Read the model definition and answer for the solid it produces. Units are mm, in the model's axes. A direction names the side the tool comes from. Round coordinates to 2 decimals unless told otherwise and drop trailing zeros. Loops run counter-clockwise (first coordinate to the right, second up) from the corner with the lowest first, then second, coordinate; pieces in that order, holes last. Notation, with made-up numbers: (56.5, -9) -> (81.5, -9) arc R22 cw to (81.5, 7) -> close; hole circle Ø7 at (66.5, -14.75). An arc over 180 degrees is marked (long way). Put each result on its own line as item: value.
from build123d import *

# Parameters (mm, degrees)
SKETCH1_W          = 30
SKETCH1_H          = 75
BASE_FLANGE1_DEPTH = 0.67
EDGE_FLANGE1_DEPTH = 75
SKETCH7_R          = 1.7
CUT_EXTRUDE1_DEPTH = 10
FILLET1_R          = 2


# Sheet-metal steps are written as plain solids
with BuildPart() as part:
    # Sketch1 → Base-Flange1 (new body)
    with BuildSketch(Plane(origin=(0, 0, 0), x_dir=(0, 0, -1), z_dir=(1, 0, 0))):
        with Locations((15, -37.5)):
            Rectangle(SKETCH1_W, SKETCH1_H)
    extrude(amount=-BASE_FLANGE1_DEPTH)

    # Edge-Flange1 section (across the edge) → Edge-Flange1 (add)
    with BuildSketch(Plane(origin=(0, -75, -30.7366), x_dir=(0, 0, 1), z_dir=(0, 1, 0))):
        with BuildLine():
            Line((-0.67, 0.7366), (-0.67, 13))
            Line((-0.67, 13), (0, 13))
            Line((0, 13), (0, 0.7366))
            ThreePointArc((0, 0.7366), (0.215745145, 0.215745145), (0.7366, 0))
            Line((0.7366, 0), (0.7366, -0.67))
            ThreePointArc((0.7366, -0.67), (-0.258016398, -0.258016398), (-0.67, 0.7366))
        make_face()
    extrude(amount=EDGE_FLANGE1_DEPTH)

    # Sketch7 → Cut-Extrude1 (cut)
    with BuildSketch(Plane(origin=(0, 0, 0), x_dir=(0, 0, -1), z_dir=(1, 0, 0))):
        with Locations((15, -60)):
            Circle(SKETCH7_R)
        with Locations((15, -15)):
            Circle(SKETCH7_R)
    extrude(amount=-CUT_EXTRUDE1_DEPTH, mode=Mode.SUBTRACT)

    # Fillet1
    fillet1_edges = [part.edges().sort_by_distance(p)[0] for p in [
        (13, -75, -31.0716),
        (13, 0, -31.0716),
        (-0.335, 0, 0),
        (-0.335, -75, 0),
    ]]
    fillet(fillet1_edges, radius=FILLET1_R)


solid = part.part
Item 1: Flat-ended cylindrical pins translate along their axes: pin 1 Ø2.5 at (y, z) = (-60, -15) entering from -X; pin 2 Ø4 at (x, y) = (8, -47) entering from +Z; pin 3 Ø5.5 at (y, z) = (-15, -15) entering from +X. Find the tip coordinate at first contact, or state that the pin passes through.
Derived:
pin 1: passes through
pin 2: stops at z = -30.74
pin 3: stops at x = 0
Item 2: The part is cut by section A-A (y = -60). Determine the outline of the cut face in (x, z).
Derived:
outline: (-0.67, -30) arc R1.41 ccw to (0.74, -31.41) -> (13, -31.41) -> (13, -30.74) -> (0.74, -30.74) arc R0.74 cw to (0, -30) -> (0, -16.7) -> (-0.67, -16.7) -> close; (-0.67, -13.3) -> (0, -13.3) -> (0, 0) -> (-0.67, 0) -> close
Item 3: The part is cut by section C-C (y = -36). Determine the outline of the cut face in (x, z).
Derived:
outline: (-0.67, -30) arc R1.41 ccw to (0.74, -31.41) -> (13, -31.41) -> (13, -30.74) -> (0.74, -30.74) arc R0.74 cw to (0, -30) -> (0, 0) -> (-0.67, 0) -> close
Item 4: Find the intervals of material crossed by line 1 along Y through (x, z) = (-0.2, -15); line 2 along X through (y, z) = (-36.5, -22); line 3 along Z through (x, y) = (11.5, -23), in increasing order.
Derived:
line 1: y = -75 to -61.7, -58.3 to -16.7, -13.3 to 0
line 2: x = -0.67 to 0
line 3: z = -31.41 to -30.74
Item 5: The part is cut by section B-B (z = -15). Determine the outline of the cut face in (x, y), then the cut area to 3 significant figures.
Derived:
outline: (-0.67, -75) -> (0, -75) -> (0, -61.7) -> (-0.67, -61.7) -> close; (-0.67, -58.3) -> (0, -58.3) -> (0, -16.7) -> (-0.67, -16.7) -> close; (-0.67, -13.3) -> (0, -13.3) -> (0, 0) -> (-0.67, 0) -> close
area: 45.7 mm^2
Item 6: Which of the six approach directions +Z, -Z, +X, -X, +Y, -Y give full straight-line access (tool end or side, diameter ignored) to faces 5 (the flat face through (7, -38, -30.737)), 6 (the flat face through (-0.4, -75, -23.2))?
Derived:
face 5: +Z, +X, +Y, -Y
face 6: +Z, -Z, +X, -X, -Y
Item 7: For a pull along Z with two mould halves and no side action, classify faces 1 (the cylindrical face through (-0.34, -0.57, -0.6)), 2 (the cylindrical face through (-0.33, -15.65, -16.57)), 3 (the flat face through (0, -37, -15)), 4 (the flat face through (7, -38, -31.407)) as pulls with the +Z half, pulls with the -Z half, needs draft (parallel to the pull), parting line crosses it, or undercut.
Derived:
face 1: pulls with the +Z half
face 2: undercut
face 3: needs draft
face 4: pulls with the -Z half
Item 8: The part is cut by section D-D (x = 2.75). Determine the outline of the cut face in (y, z), then the cut area to 4 significant figures.
Derived:
outline: (-75, -31.41) -> (0, -31.41) -> (0, -30.74) -> (-75, -30.74) -> close
area: 50.25 mm^2
